The listing builds one solid part. Answer for the finished solid, in the listing's coordinates (mm). Round coordinates to 2 decimals unless told otherwise and drop trailing zeros. Loops run counter-clockwise (first coordinate to the right, second up) from the corner with the lowest first, then second, coordinate; pieces in that order, holes last. Notation, with made-up numbers: (-36, 69) - (-32, 69) arc R30 cw to (-32, 98) - close; hole circle Ø2 at (54.25, 25). An arc over 180 degrees is marked (long way). One line per question, with ' | ' between items. Start each with the question number.
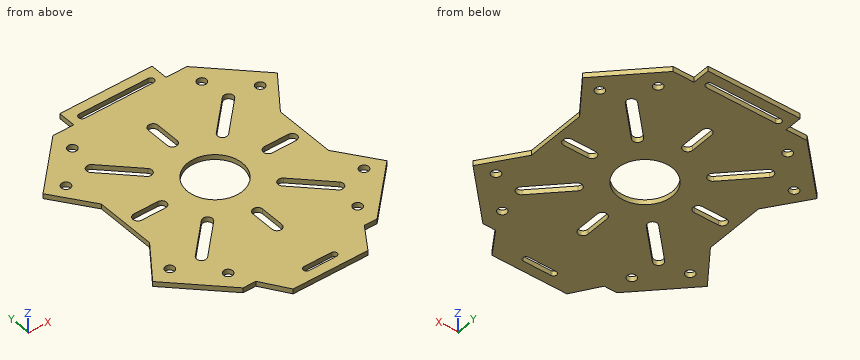
from build123d import *

# Parameters (mm, degrees)
F0_R     = 1.5
F0_R_2   = 9
F1_DEPTH = 1.6256


with BuildPart() as f1:
    # F0 (on Top) → F1 (new body)
    with BuildSketch(Plane.XY):
        Polygon((-29.337, 9.8425), (-29.337, -9.8425), (-38.3921, -22.404234), (-21.959734, -38.8366), (-17.78, -38.8366), (-12.2555, -47.1932), (0, -47.1932), (12.2555, -47.1932), (17.78, -38.8366), (21.959734, -38.8366), (38.3921, -22.404234), (29.337, -9.8425), (29.337, 9.8425), (38.3921, 22.404234), (21.959734, 38.8366), (15.113, 38.8366), (15.113, 44.5516), (0, 44.5516), (-15.113, 44.5516), (-15.113, 38.8366), (-21.959734, 38.8366), (-38.3921, 22.404234), align=None)
        with Locations((-21.213203, -31.819805)):
            Circle(F0_R, mode=Mode.SUBTRACT)
        with Locations((-31.819805, -21.213203)):
            Circle(F0_R, mode=Mode.SUBTRACT)
        with BuildLine():
            ThreePointArc((-21.354625, -23.599689), (-23.599689, -23.599689), (-23.599689, -21.354625))
            Line((-23.599689, -21.354625), (-13.470384, -11.22532))
            ThreePointArc((-13.470384, -11.22532), (-11.22532, -11.22532), (-11.22532, -13.470384))
            Line((-11.22532, -13.470384), (-21.354625, -23.599689))
        make_face(mode=Mode.SUBTRACT)
        with BuildLine():
            ThreePointArc((-4.5085, -43.9928), (-5.5245, -42.9768), (-4.5085, -41.9608))
            Line((-4.5085, -41.9608), (4.5085, -41.9608))
            ThreePointArc((4.5085, -41.9608), (5.5245, -42.9768), (4.5085, -43.9928))
            Line((4.5085, -43.9928), (-4.5085, -43.9928))
        make_face(mode=Mode.SUBTRACT)
        with Locations((21.213203, -31.819805)):
            Circle(F0_R, mode=Mode.SUBTRACT)
        with BuildLine():
            Line((1.5875, -17.4625), (1.5875, -25.2875))
            ThreePointArc((1.5875, -25.2875), (0, -26.875), (-1.5875, -25.2875))
            Line((-1.5875, -25.2875), (-1.5875, -17.4625))
            ThreePointArc((-1.5875, -17.4625), (0, -15.875), (1.5875, -17.4625))
        make_face(mode=Mode.SUBTRACT)
        with BuildLine():
            ThreePointArc((23.599689, -21.354625), (23.599689, -23.599689), (21.354625, -23.599689))
            Line((21.354625, -23.599689), (11.22532, -13.470384))
            ThreePointArc((11.22532, -13.470384), (11.22532, -11.22532), (13.470384, -11.22532))
            Line((13.470384, -11.22532), (23.599689, -21.354625))
        make_face(mode=Mode.SUBTRACT)
        with Locations((31.819805, -21.213203)):
            Circle(F0_R, mode=Mode.SUBTRACT)
        with BuildLine():
            Line((-17.4625, -1.5875), (-25.2875, -1.5875))
            ThreePointArc((-25.2875, -1.5875), (-26.875, 0), (-25.2875, 1.5875))
            Line((-25.2875, 1.5875), (-17.4625, 1.5875))
            ThreePointArc((-17.4625, 1.5875), (-15.875, 0), (-17.4625, -1.5875))
        make_face(mode=Mode.SUBTRACT)
        with Locations((-31.819805, 21.213203)):
            Circle(F0_R, mode=Mode.SUBTRACT)
        with BuildLine():
            Line((-13.470384, 11.22532), (-23.599689, 21.354625))
            ThreePointArc((-23.599689, 21.354625), (-23.599689, 23.599689), (-21.354625, 23.599689))
            Line((-21.354625, 23.599689), (-11.22532, 13.470384))
            ThreePointArc((-11.22532, 13.470384), (-11.22532, 11.22532), (-13.470384, 11.22532))
        make_face(mode=Mode.SUBTRACT)
        with Locations((-21.213203, 31.819805)):
            Circle(F0_R, mode=Mode.SUBTRACT)
        Circle(F0_R_2, mode=Mode.SUBTRACT)
        with BuildLine():
            Line((-1.5875, 17.4625), (-1.5875, 25.2875))
            ThreePointArc((-1.5875, 25.2875), (0, 26.875), (1.5875, 25.2875))
            Line((1.5875, 25.2875), (1.5875, 17.4625))
            ThreePointArc((1.5875, 17.4625), (0, 15.875), (-1.5875, 17.4625))
        make_face(mode=Mode.SUBTRACT)
        with BuildLine():
            ThreePointArc((21.354625, 23.599689), (23.599689, 23.599689), (23.599689, 21.354625))
            Line((23.599689, 21.354625), (13.470384, 11.22532))
            ThreePointArc((13.470384, 11.22532), (11.22532, 11.22532), (11.22532, 13.470384))
            Line((11.22532, 13.470384), (21.354625, 23.599689))
        make_face(mode=Mode.SUBTRACT)
        with BuildLine():
            Line((17.4625, 1.5875), (25.2875, 1.5875))
            ThreePointArc((25.2875, 1.5875), (26.875, 0), (25.2875, -1.5875))
            Line((25.2875, -1.5875), (17.4625, -1.5875))
            ThreePointArc((17.4625, -1.5875), (15.875, 0), (17.4625, 1.5875))
        make_face(mode=Mode.SUBTRACT)
        with Locations((31.819805, 21.213203)):
            Circle(F0_R, mode=Mode.SUBTRACT)
        with BuildLine():
            ThreePointArc((-11.2903, 39.1668), (-12.3825, 40.259), (-11.2903, 41.3512))
            Line((-11.2903, 41.3512), (11.2903, 41.3512))
            ThreePointArc((11.2903, 41.3512), (12.3825, 40.259), (11.2903, 39.1668))
            Line((11.2903, 39.1668), (-11.2903, 39.1668))
        make_face(mode=Mode.SUBTRACT)
        with Locations((21.213203, 31.819805)):
            Circle(F0_R, mode=Mode.SUBTRACT)
    extrude(amount=F1_DEPTH)


solid = f1.part
(1) Find section C-C on z = 1.35. Count the separate pieces of the cut face and the enclosed holes in it, plus the area to 3 significant figures.
(2) Find section B-B on x = 0. Write down the section's boundary in (y, z) (3 decimals).
(3) Consider L1, parallel to Y at x = 2, z = 0.95; L2, parallel to X at y = 20.5, z = 0.25; L3, parallel to Y at x = -1, z = 1.55. Determine where each line is inside the solid, lowest interval first.
(4) Find section D-D on x = 28. Write down the section's boundary in (y, z).
(5) Find section A-A on y = 0. Write down the section's boundary in (x, z) (3 decimals).
(6) Each of these flat-tipped pins is pushed along its axis until it touches: P1, Ø0.8, axis at x = -22.5, z = 1, coming from the -Y side; P2, Ø0.5, axis at y = -22, z = 0.5, coming from the -X side. Where does it stop, or does it pass through?
Answer below:
1) separate pieces: 1 | enclosed holes: 19 | area: 4,530 mm2
2) outline: (-47.193, 0) - (-43.993, 0) - (-43.993, 1.626) - (-47.193, 1.626) - close; (-41.961, 0) - (-26.875, 0) - (-26.875, 1.626) - (-41.961, 1.626) - close; (-15.875, 0) - (-9, 0) - (-9, 1.626) - (-15.875, 1.626) - close; (9, 0) - (15.875, 0) - (15.875, 1.626) - (9, 1.626) - close; (26.875, 0) - (39.167, 0) - (39.167, 1.626) - (26.875, 1.626) - close; (41.351, 0) - (44.552, 0) - (44.552, 1.626) - (41.351, 1.626) - close
3) L1: -47.19 to -43.99, -41.96 to -8.77, 8.77 to 39.17, 41.35 to 44.55 | L2: -37.02 to -33.14, -30.5 to -22.75, -18.25 to -1.59, 1.59 to 18.25, 22.75 to 30.5, 33.14 to 37.02 | L3: -47.19 to -43.99, -41.96 to -26.52, -16.23 to -8.94, 8.94 to 16.23, 26.52 to 39.17, 41.35 to 44.55
4) outline: (-32.8, 0) - (32.8, 0) - (32.8, 1.63) - (-32.8, 1.63) - close
5) outline: (-29.337, 0) - (-26.875, 0) - (-26.875, 1.626) - (-29.337, 1.626) - close; (-15.875, 0) - (-9, 0) - (-9, 1.626) - (-15.875, 1.626) - close; (9, 0) - (15.875, 0) - (15.875, 1.626) - (9, 1.626) - close; (26.875, 0) - (29.337, 0) - (29.337, 1.626) - (26.875, 1.626) - close
6) P1: y = -38.7 | P2: x = -38.28
